```python
from build123d import *

# Parameters (mm, degrees)
SKETCH_1_R          = 7
EXTRUDE_1_DEPTH     = 3
SKETCH_2_R          = 4
EXTRUDE_2_DEPTH     = 23
SKETCH_3_OUTSIDE_W  = 22.536
SKETCH_3_OUTSIDE_H  = 22.536
SKETCH_3_OUTSIDE_R  = 3
CUT_EXTRUDE_1_DEPTH = 2
CHAMFER_1_SIZE      = 0.5


with BuildPart() as part:
    # 草图1 → 凸台-拉伸1 (new body)
    with BuildSketch(Plane.XY):
        Circle(SKETCH_1_R)
    extrude(amount=EXTRUDE_1_DEPTH)

    # 草图2 → 凸台-拉伸2 (add)
    with BuildSketch(Plane.XY.offset(3)):
        Circle(SKETCH_2_R)
    extrude(amount=EXTRUDE_2_DEPTH)

    # 草图3 outside → 切除-拉伸1 (cut)
    with BuildSketch(Plane.XY.offset(3)):
        Rectangle(SKETCH_3_OUTSIDE_W, SKETCH_3_OUTSIDE_H)
        Circle(SKETCH_3_OUTSIDE_R, mode=Mode.SUBTRACT)
    extrude(amount=CUT_EXTRUDE_1_DEPTH, mode=Mode.SUBTRACT)

    # 倒角1
    chamfer_1_edges = [part.edges().sort_by_distance(p)[0] for p in [
        (-7, 0, 0),
        (-4, 0, 26),
    ]]
    chamfer(chamfer_1_edges, length=CHAMFER_1_SIZE)

    # 草图4 → 切除-旋转1 (revolve, cut)
    with BuildSketch(Plane(origin=(0, 0, 0), x_dir=(0, 0, -1), z_dir=(1, 0, 0)), mode=Mode.PRIVATE) as cut_revolve_1_sk:
        Polygon((-18.5, 2), (-16.5, 4), (-18.5, 4), align=None)
    revolve(cut_revolve_1_sk.sketch.rotate(Axis((0, 6.943953148, 18.5), (0, -1, 0)), 180), axis=Axis((0, 6.943953148, 18.5), (0, -1, 0)), mode=Mode.SUBTRACT)


solid = part.part
```
Model file for the job. Use its own axes, mm. A direction names the side the tool comes from. Give positions to 0.01 mm unless a question says otherwise; leave off trailing zeros. Write each loop counter-clockwise with the first axis right and the second up, starting at its lowest first coordinate (ties: lowest second). Pieces come first, ordered by that corner, then holes. Notation, with made-up numbers: M -27,47 L -20,47 A16 ccw -20,54 Z; hole C -7.5,24 d9. An arc over 180 degrees is marked long. Use a Markdown table: item, result.
1) Drill centre lines: line 1 (Z direction, x = -1, y = 5.75); line 2 (Z direction, x = 2.75, y = 2.5); line 3 (X direction, y = -1.75, z = 20). Where is each one in solid material? Low to high. Write a range as from..to.
Responses:
| item | result |
|---|---|
| line 1 | z = 0..3 |
| line 2 | z = 0..3, 5..25.78 |
| line 3 | x = -3.6..3.6 |
2) Cut at A-A (y = 0). List the corners of the cut face in (x, z).
Responses:
| item | result |
|---|---|
| outline | M -7,0.5 L -6.5,0 L 6.5,0 L 7,0.5 L 7,3 L 3,3 L 3,5 L 4,5 L 4,25.5 L 3.5,26 L -3.5,26 L -4,25.5 L -4,5 L -3,5 L -3,3 L -7,3 Z |
3) Pull direction Z, two halves, no side cores. Call faces 4 (the flat face through (1, 3, 5)), 5 (the flat face through (0, 0, 0)), 6 (the cylindrical face through (6.466, -2.681, 1.732)): +Z half, -Z half, draft (parallel to the pull), parting line (faces both ways), or undercut.
Responses:
| item | result |
|---|---|
| face 4 | undercut |
| face 5 | -Z half |
| face 6 | draft |
4) Tool access for faces 1 (the flat face through (0, 0, 26)), 2 (the cylindrical face through (-3, 0, 4)), 3 (the cylindrical face through (-0.867, -3.905, 15.106)): list every direction of +Z, -Z, +X, -X, +Y, -Y with a clear straight run to the whole face (end or side of a thin tool).
Responses:
| item | result |
|---|---|
| face 1 | +Z, +X, -X, +Y, -Y |
| face 2 | none |
| face 3 | +Z |
5) Cut at B-B (z = 10). List the corners of the cut face in (x, y), and give its area (3 significant figures).
Responses:
| item | result |
|---|---|
| outline | C 0,0 d8 |
| area | 50.3 mm2 |
6) Pin check, flat tips, straight feed: pin 1 (6 mm diameter, centred on x = -4, z = 18.5, fed in from -Y); pin 2 (8 mm diameter, centred on x = -4, z = 11.5, fed in from +Y); pin 3 (4 mm diameter, centred on x = -5, y = 4, fed in from +Z). Stop position of each tip, or through.
Responses:
| item | result |
|---|---|
| pin 1 | stops at y = -3.87 |
| pin 2 | stops at y = 4 |
| pin 3 | stops at z = 3 |
